Design review of the part built by this model. Coordinates are the model's own, in mm. Round coordinates to 2 decimals unless told otherwise and drop trailing zeros. Order: outer loops, then holes, each group sorted by start corner. A loop starts at its lowest first (then second) coordinate and runs counter-clockwise, first axis right, second up. Notation, with made-up numbers: M 66,-1.5 L 125,-1.5 A36 ccw 125,37.5 Z; hole C -25,4 d1. An arc over 180 degrees is marked long. Use a Markdown table: item, result. Add a question column.
(1) For pin 1 (1 mm diameter, centred on x = -0.5, y = 0, fed in from +Z); pin 2 (1 mm diameter, centred on y = -1.5, z = -117, fed in from +X); pin 3 (1 mm diameter, centred on x = 0.5, y = 0, fed in from -Z), all flat-tipped, find the tip position at first contact; note any pin that passes through.
(2) To check wall thickness, follow probe 1 along Y at (x, z) = (0.5, -108); probe 2 along Z at (x, y) = (1.5, 0); probe 3 along Y at (x, z) = (-2.5, -10). State the ranges of each line that lie inside material, in increasing order. Write a range as from..to.
(3) Take a section at C-C (z = -65). Write out the cut boundary in (x, y).
(4) Take a section at A-A (x = 0). Write out the cut boundary in (y, z), then the cut area to 3 significant figures.
```python
from build123d import *

# Parameters (mm, degrees)
SKETCH29_R         = 1.65
CUT_EXTRUDE1_DEPTH = 10
CUT_EXTRUDE2_START = -12
SKETCH30_R         = 1.65
CUT_EXTRUDE2_DEPTH = 12


with BuildPart() as part:
    # Sketch22 → Revolve1 (revolve)
    with BuildSketch(Plane(origin=(0, 0, 0), x_dir=(0, 0, -1), z_dir=(1, 0, 0)), mode=Mode.PRIVATE) as revolve1_sk:
        Polygon((-148.5, 0), (-148.5, 3.2), (-147.939833969, 4), (147.939833969, 4), (148.5, 3.2), (148.5, 0), align=None)
    revolve(revolve1_sk.sketch.rotate(Axis((0, 0, -148.5), (0, 0, -1)), 180), axis=Axis((0, 0, -148.5), (0, 0, -1)))

    # Sketch29 → Cut-Extrude1 (cut)
    with BuildSketch(Plane.XY.offset(-148.5)):
        Circle(SKETCH29_R)
    extrude(amount=CUT_EXTRUDE1_DEPTH, mode=Mode.SUBTRACT)

    # Sketch30 → Cut-Extrude2 (cut)
    with BuildSketch(Plane.XY.offset(148.5).offset(CUT_EXTRUDE2_START)):
        Circle(SKETCH30_R)
    extrude(amount=CUT_EXTRUDE2_DEPTH, mode=Mode.SUBTRACT)


solid = part.part
```
Verdict:
| question | item | result |
|---|---|---|
| 1 | pin 1 | stops at z = 136.5 |
| 1 | pin 2 | stops at x = 3.87 |
| 1 | pin 3 | stops at z = -138.5 |
| 2 | probe 1 | y = -3.97..3.97 |
| 2 | probe 2 | z = -138.5..136.5 |
| 2 | probe 3 | y = -3.12..3.12 |
| 3 | outline | C 0,0 d8 |
| 4 | outline | M -4,-147.94 L -3.2,-148.5 L -1.65,-148.5 L -1.65,-138.5 L 1.65,-138.5 L 1.65,-148.5 L 3.2,-148.5 L 4,-147.94 L 4,147.94 L 3.2,148.5 L 1.65,148.5 L 1.65,136.5 L -1.65,136.5 L -1.65,148.5 L -3.2,148.5 L -4,147.94 Z |
| 4 | area | 2,300 mm^2 |
